The figure shows three views and two pictorial views of one solid part (mm, origin at its lowest corner). Answer the questions. A direction names the side the tool comes from. Coordinates: 2 decimals unless noted, no trailing zeros. Loops run counter-clockwise (first coordinate to the right, second up) from the corner with the lowest first, then second, coordinate; pieces in that order, holes last. Notation, with made-up numbers: (19.25, -16) - (64.25, -16) arc R33 ccw to (64.25, 22) - close; hole circle Ø10 at (4, 87). An arc over 180 degrees is marked (long way). Write each question's results on one line, items separated by ' | '. Start each with the question number.
Item 1: Section A-A, the plane x = 8.5 is taken. Write down the section's boundary in (y, z).
Item 2: A tool of negligible diameter and unlimited length cuts with its end or side. For the marked faces 5 and 6, from which of +Z, -Z, +X, -X, +Y, -Y can it reach the whole face along a straight path? Write none if from no direction.
Item 3: Each of these flat-tipped pins is pushed along its axis until it touches: pin 1 Ø1.1 at (x, z) = (0.5, 18.5) entering from +Y; pin 2 Ø5 at (x, z) = (4, 17) entering from +Y; pin 3 Ø4.5 at (x, y) = (7.5, 5) entering from -Z. Where does it stop, or does it pass through?
Item 4: Section D-D, the plane x = 11 is taken. Write down the section's boundary in (y, z), plus the area to 3 significant figures.
Item 5: Section B-B, the plane y = 6 is taken. Write down the section's boundary in (x, z), plus the area to 3 significant figures.
Item 6: For a pull along X with two mould halves and no side action, classify the marked faces 1, 2, 3 and 4 as +X half, -X half, draft (parallel to the pull), parting line (faces both ways), or undercut.
Item 7: Consider probe 1 along X at (y, z) = (6, 32.8); probe 2 along X at (y, z) = (6.5, 4.5); probe 3 along Z at (x, y) = (12, 8.75). Determine where each line is inside the solid, lowest interval first. Write a range as [from, to].
Item 8: Section C-C, the plane z = 4 is taken. Write down the section's boundary in (x, y).
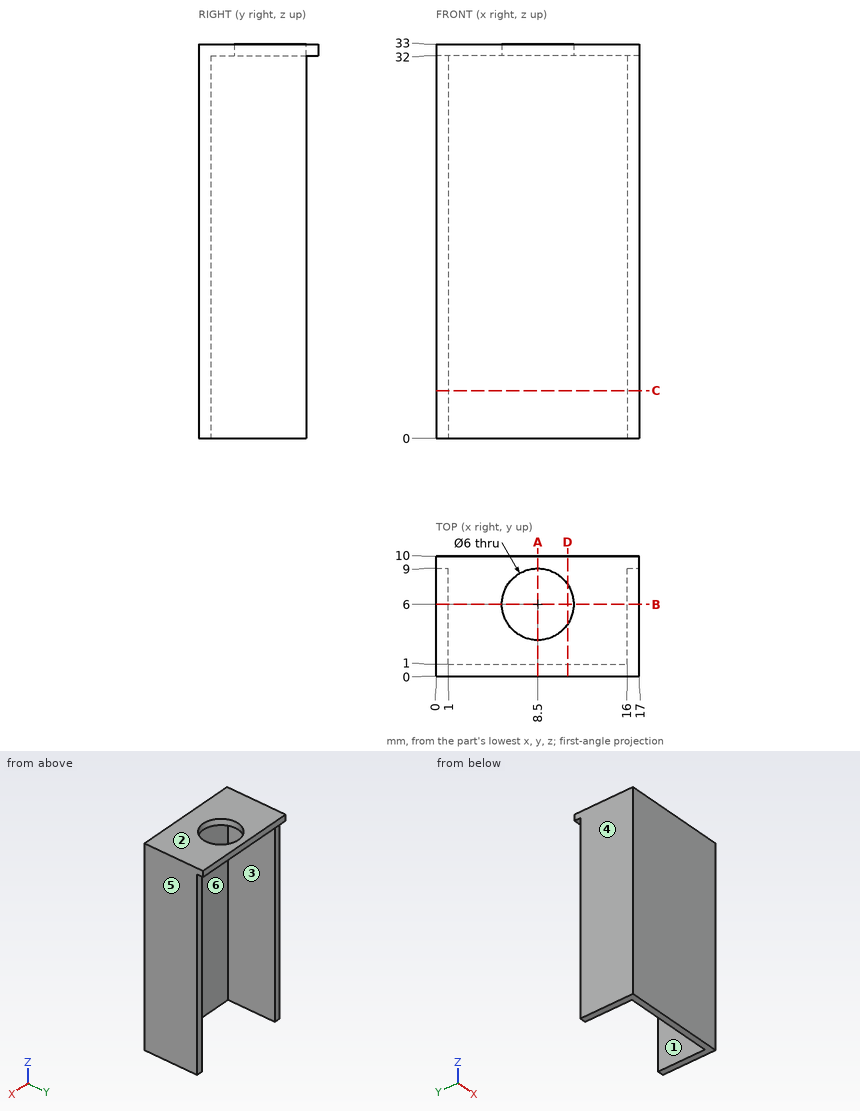
Answer key:
1) outline: (0, 0) - (1, 0) - (1, 32) - (3, 32) - (3, 33) - (0, 33) - close; (9, 32) - (10, 32) - (10, 33) - (9, 33) - close
2) face 5: +Z, -Z, +X, +Y, -Y | face 6: -Z, +Y
3) pin 1: stops at y = 9 | pin 2: stops at y = 1 | pin 3: stops at z = 32
4) outline: (0, 0) - (1, 0) - (1, 32) - (4.34, 32) - (4.34, 33) - (0, 33) - close; (7.66, 32) - (10, 32) - (10, 33) - (7.66, 33) - close | area: 38.7 mm^2
5) outline: (0, 0) - (1, 0) - (1, 32) - (5.5, 32) - (5.5, 33) - (0, 33) - close; (11.5, 32) - (16, 32) - (16, 0) - (17, 0) - (17, 33) - (11.5, 33) - close | area: 75.0 mm^2
6) face 1: undercut | face 2: draft | face 3: undercut | face 4: -X half
7) probe 1: x = [0, 5.5], [11.5, 17] | probe 2: x = [0, 1], [16, 17] | probe 3: z = [32, 33]
8) outline: (0, 0) - (17, 0) - (17, 9) - (16, 9) - (16, 1) - (1, 1) - (1, 9) - (0, 9) - close
